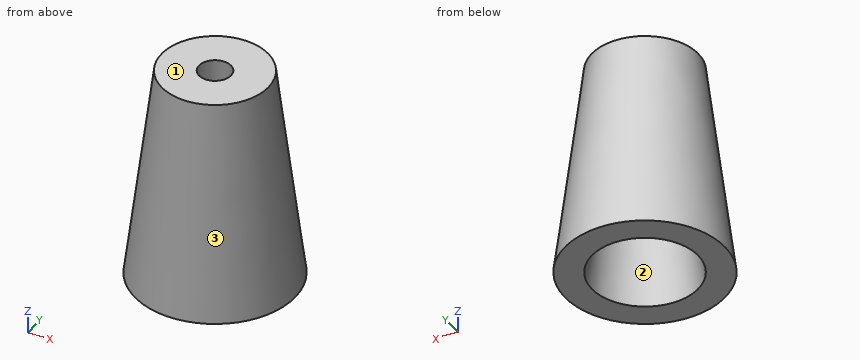
```python
from build123d import *

# Parameters (mm, degrees)
F0_R     = 7.5
F2_R     = 5
F4_T     = -2.5
F5_R     = 1.5
F6_DEPTH = 25


with BuildPart() as f3:
    # F0 (on Top) → F3 section 0
    with BuildSketch(Plane.XY):
        Circle(F0_R)
    # F2 (on offset) → F3 section 1
    with BuildSketch(Plane.XY.offset(20)):
        Circle(F2_R)
    loft()

    # F4
    f4_openings = [f3.faces().sort_by_distance(p)[0] for p in [
        (0, 0, 0),
    ]]
    offset(amount=F4_T, openings=f4_openings, kind=Kind.INTERSECTION)

    # F5 (on face) → F6 (cut)
    with BuildSketch(Plane.XY.offset(20)):
        Circle(F5_R)
    extrude(amount=-F6_DEPTH, mode=Mode.SUBTRACT)


solid = f3.part
```
CAD build for the part. Positions are in the model's coordinates, mm. Face numbers are marked on the shaded views. Coordinates: 2 decimals unless noted, no trailing zeros. Loops run counter-clockwise (first coordinate to the right, second up) from the corner with the lowest first, then second, coordinate; pieces in that order, holes last. Notation, with made-up numbers: (65.5, -38.5) - (70.5, -38.5) arc R13 cw to (70.5, -18.5) - close; hole circle Ø4 at (-1.5, 61). An arc over 180 degrees is marked (long way). Use CSV: the item, a comma, the result in double quotes. Start each with the question number.
Q1. Cut at A-A, the plane x = 0. List the corners of the cut face in (y, z).
Q2. Two-plate mould, pull along Y, no slides. Class the marked faces 1, 2 and 3: +Y half, -Y half, draft (parallel to the pull), parting line (faces both ways), or undercut.
Q3. Probe probe 1 along Z at (x, y) = (1.25, -2); probe 2 along X at (y, z) = (-2.75, 13.75); probe 3 along X at (y, z) = (-0.5, 14.25). List the from-to ranges inside material, lowest first. Write a range as from..to.
Q4. Cut at C-C, the plane z = 14. List the corners of the cut face in (x, y), then the cut area to 3 significant figures.
Q5. Cut at B-B, the plane z = 16.75. List the corners of the cut face in (x, y), then the cut area to 3 significant figures.
Q6. Drop flat-ended pins along their axis: P1, Ø8, axis at y = 3, z = 12.5, coming from the +X side; P2, Ø3, axis at x = -2, z = 16, coming from the -Y side; P3, Ø6, axis at x = 2.5, z = 7.5, coming from the +Y side. Give the stop position or say it passes through.
Here are the results:
1,outline,"(-7.5, 0) - (-4.98, 0) - (-2.79, 17.5) - (-1.5, 17.5) - (-1.5, 20) - (-5, 20) - close; (1.5, 17.5) - (2.79, 17.5) - (4.98, 0) - (7.5, 0) - (5, 20) - (1.5, 20) - close"
2,face 1,"draft"
2,face 2,"undercut"
2,face 3,"parting line"
3,probe 1,"17.5..20"
3,probe 2,"-5.09..-1.75, 1.75..5.09"
3,probe 3,"-5.7..-3.16, 3.16..5.7"
4,outline,"circle Ø11.5 at (0, 0); hole circle Ø6.46 at (0, 0)"
4,area,"71.1 mm2"
5,outline,"circle Ø10.81 at (0, 0); hole circle Ø5.77 at (0, 0)"
5,area,"65.6 mm2"
6,P1,"x = 6.31"
6,P2,"y = -5.56"
6,P3,"y = 6.83"
